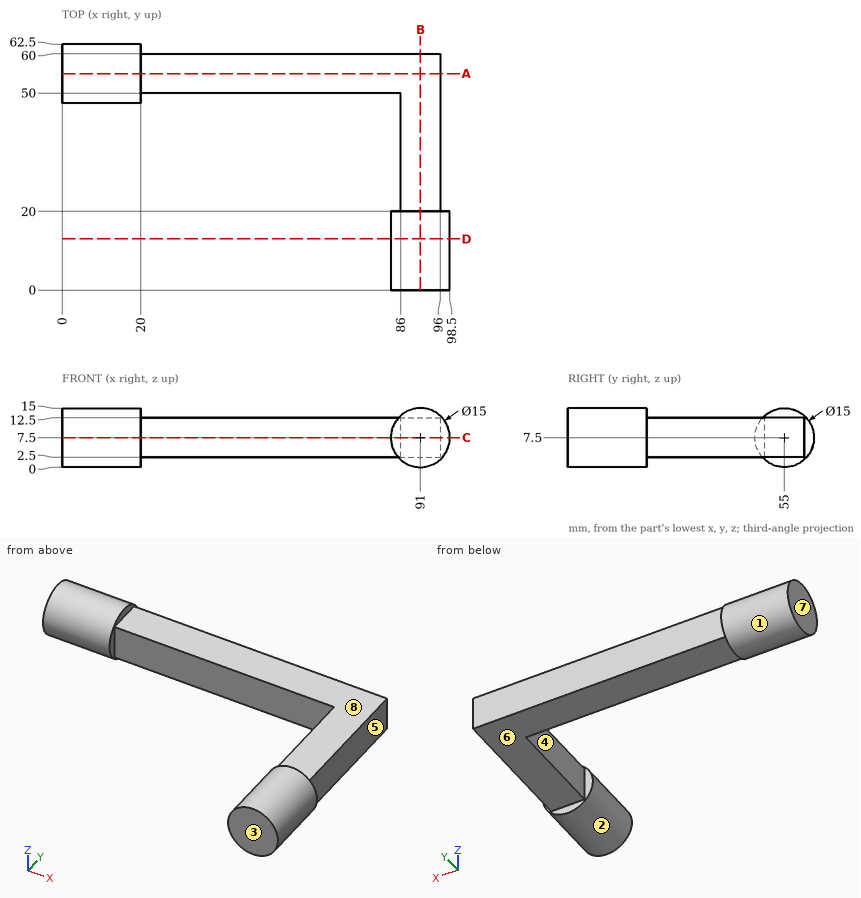
Answer from the drawing. Dimensions are ordinates in mm from the lowest x, y and z of the part. A direction names the side the tool comes from. Round coordinates to 2 decimals unless told otherwise and drop trailing zeros. Order: outer loops, then holes, each group sorted by start corner. A loop starts at its lowest first (then second) coordinate and runs counter-clockwise, first axis right, second up. Notation, with made-up numbers: (-13, -25.5) -> (4, -25.5) arc R15 ccw to (4, 2.5) -> close; hole circle Ø8 at (5.25, 21). An arc over 180 degrees is marked (long way). Answer as CSV lines item,"result".
Q1. A cutting plane is placed at A-A on y = 55. Determine the outline of the cut face in (x, z), plus the area to 3 significant figures.
Computed values:
outline,"(0, 0) -> (20, 0) -> (20, 2.5) -> (96, 2.5) -> (96, 12.5) -> (20, 12.5) -> (20, 15) -> (0, 15) -> close"
area,"1,060 mm^2"
Q2. Consider line 1 (Y direction, x = 74.5, z = 7); line 2 (Y direction, x = 15, z = 7.25); line 3 (X direction, y = 35.5, z = 9). Determine where each line is inside the solid, lowest interval first. Write a range as from..to.
Computed values:
line 1,"y = 50..60"
line 2,"y = 47.5..62.5"
line 3,"x = 86..96"
Q3. A cutting plane is placed at C-C on z = 7.5. Determine the outline of the cut face in (x, y).
Computed values:
outline,"(0, 47.5) -> (20, 47.5) -> (20, 50) -> (86, 50) -> (86, 20) -> (83.5, 20) -> (83.5, 0) -> (98.5, 0) -> (98.5, 20) -> (96, 20) -> (96, 60) -> (20, 60) -> (20, 62.5) -> (0, 62.5) -> close"
Q4. A cutting plane is placed at B-B on x = 91. Determine the outline of the cut face in (y, z).
Computed values:
outline,"(0, 0) -> (20, 0) -> (20, 2.5) -> (60, 2.5) -> (60, 12.5) -> (20, 12.5) -> (20, 15) -> (0, 15) -> close"
Q5. Which of the six approach directions +Z, -Z, +X, -X, +Y, -Y give full straight-line access (tool end or side, diameter ignored) to the marked faces 5, 6, 7 and 8?
Computed values:
face 5,"+Z, -Z, +X, +Y"
face 6,"-Z, +X, +Y"
face 7,"+Z, -Z, -X, +Y, -Y"
face 8,"+Z, +X, +Y"
Q6. Given pin 1 (3 mm diameter, centred on x = 69.5, z = 6.5, fed in from +Y); pin 2 (3 mm diameter, centred on y = 33.5, z = 6, fed in from -X); pin 3 (1.5 mm diameter, centred on y = 39.5, z = 5, fed in from +X); pin 4 (1.5 mm diameter, centred on x = 62, y = 47.5, fed in from -Z), each flat-ended and moving along its own axis, determine where each tip first touches the part or whether it passes through.
Computed values:
pin 1,"stops at y = 60"
pin 2,"stops at x = 86"
pin 3,"stops at x = 96"
pin 4,"passes through"
Q7. For a pull along Y with two mould halves and no side action, classify the marked faces 1, 2, 3 and 4 as +Y half, -Y half, draft (parallel to the pull), parting line (faces both ways), or undercut.
Computed values:
face 1,"parting line"
face 2,"draft"
face 3,"-Y half"
face 4,"undercut"
Q8. A cutting plane is placed at D-D on y = 13. Determine the outline of the cut face in (x, z).
Computed values:
outline,"circle Ø15 at (91, 7.5)"
